Can you work these out from the drawing? Everything is in mm from the part's minimum corner. Coordinates: 2 decimals unless noted, no trailing zeros. Loops run counter-clockwise (first coordinate to the right, second up) from the corner with the lowest first, then second, coordinate; pieces in that order, holes last. Notation, with made-up numbers: (38.5, -30) - (45.5, -30) arc R27 ccw to (45.5, -12) - close; hole circle Ø10 at (85, 58). An arc over 180 degrees is marked (long way). One line per question, with ' | ' between items. Start each with the question number.
1. I want a section at D-D, the plane x = 114.2. Write out the boundary of the cut face in (y, z).
2. I'm going to push flat-ended pins straight in: P1, Ø2, axis at x = 96, z = 14.5, coming from the +Y side; P2, Ø2, axis at x = 18, y = 6.5, coming from the +Z side; P3, Ø5, axis at x = 5, z = 53, coming from the +Y side. Where does each tip first touch, or does it pass through?
3. I want a section at A-A, the plane y = 2.5. Write out the boundary of the cut face in (x, z), then the cut area to 3 significant figures.
4. I want a section at C-C, the plane z = 52.2. Write out the boundary of the cut face in (x, y), then the cut area to 3 significant figures.
5. We'd pull the mould along X, two halves only. Please class the marked faces 1 and 2: pulls with the +X half, pulls with the -X half, needs draft (parallel to the pull), parting line crosses it, or undercut.
6. I want a section at B-B, the plane z = 3.2. Write out the boundary of the cut face in (x, y).
7. Please list where these lines run through material, in increasing order: L1, parallel to Z at x = 3.2, y = 0.4; L2, parallel to X at y = 0.6, z = 3.2; L3, parallel to X at y = 0.4, z = 52.2. Write a range as [from, to].
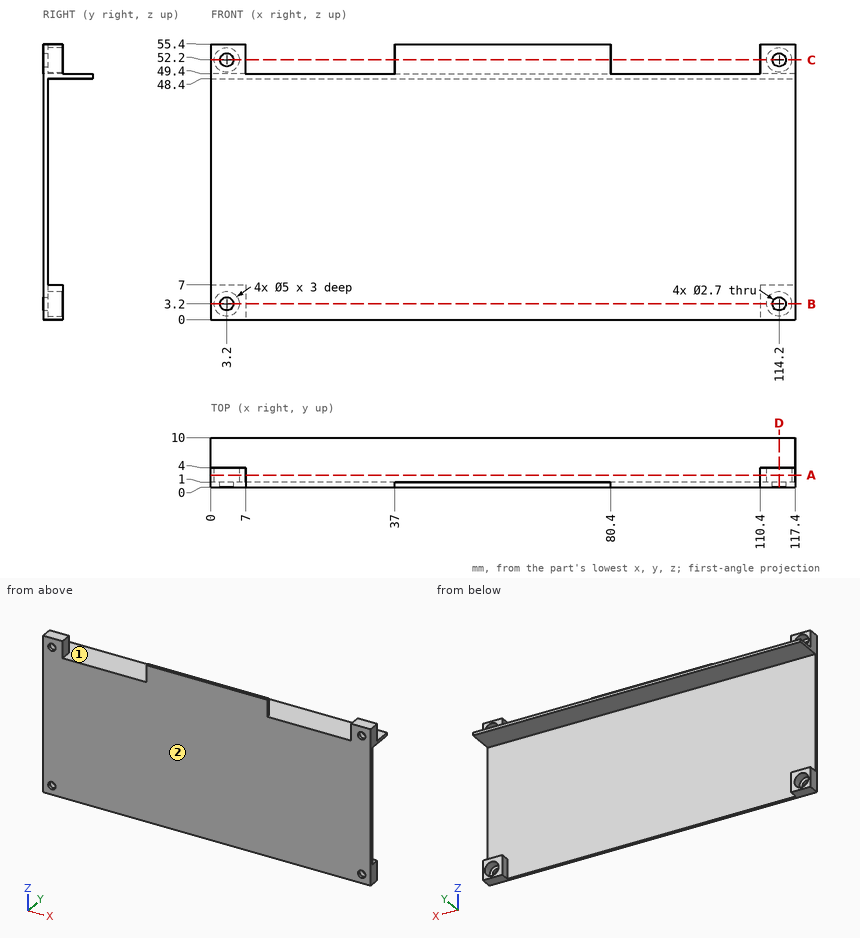
Results are:
1) outline: (0, 0) - (4, 0) - (4, 0.7) - (1, 0.7) - (1, 1.85) - (0, 1.85) - close; (0, 4.55) - (1, 4.55) - (1, 5.7) - (4, 5.7) - (4, 7) - (1, 7) - (1, 48.4) - (10, 48.4) - (10, 49.4) - (4, 49.4) - (4, 49.7) - (1, 49.7) - (1, 50.85) - (0, 50.85) - close; (0, 53.55) - (1, 53.55) - (1, 54.7) - (4, 54.7) - (4, 55.4) - (0, 55.4) - close
2) P1: stops at y = 1 | P2: stops at z = 49.4 | P3: stops at y = 4
3) outline: (0, 0) - (7, 0) - (7, 7) - (0, 7) - close; (0, 48.4) - (117.4, 48.4) - (117.4, 55.4) - (110.4, 55.4) - (110.4, 49.4) - (7, 49.4) - (7, 55.4) - (0, 55.4) - close; (110.4, 0) - (117.4, 0) - (117.4, 7) - (110.4, 7) - close; hole circle Ø5 at (3.2, 3.2); hole circle Ø5 at (3.2, 52.2); hole circle Ø5 at (114.2, 3.2); hole circle Ø5 at (114.2, 52.2) | area: 221 mm2
4) outline: (0, 0) - (1.85, 0) - (1.85, 1) - (0.7, 1) - (0.7, 4) - (0, 4) - close; (4.55, 0) - (7, 0) - (7, 4) - (5.7, 4) - (5.7, 1) - (4.55, 1) - close; (37, 0) - (80.4, 0) - (80.4, 1) - (37, 1) - close; (110.4, 0) - (112.85, 0) - (112.85, 1) - (111.7, 1) - (111.7, 4) - (110.4, 4) - close; (115.55, 0) - (117.4, 0) - (117.4, 4) - (116.7, 4) - (116.7, 1) - (115.55, 1) - close | area: 64.0 mm2
5) face 1: undercut | face 2: needs draft
6) outline: (0, 0) - (1.85, 0) - (1.85, 1) - (0.7, 1) - (0.7, 4) - (0, 4) - close; (4.55, 0) - (112.85, 0) - (112.85, 1) - (111.7, 1) - (111.7, 4) - (110.4, 4) - (110.4, 1) - (7, 1) - (7, 4) - (5.7, 4) - (5.7, 1) - (4.55, 1) - close; (115.55, 0) - (117.4, 0) - (117.4, 4) - (116.7, 4) - (116.7, 1) - (115.55, 1) - close
7) L1: z = [0, 1.85], [4.55, 50.85], [53.55, 55.4] | L2: x = [0, 1.85], [4.55, 112.85], [115.55, 117.4] | L3: x = [0, 1.85], [4.55, 7], [37, 80.4], [110.4, 112.85], [115.55, 117.4]
